The listing builds one solid part. Answer for the finished solid, in the listing's coordinates (mm). Face numbers are marked on the shaded views. A direction names the side the tool comes from. Give positions to 0.01 mm unless a question says otherwise; leave off trailing zeros. Loops run counter-clockwise (first coordinate to the right, second up) from the corner with the lowest first, then second, coordinate; pieces in that order, holes last. Notation, with made-up numbers: M 88,31.5 L 115,31.5 A14 cw 115,49.5 Z; hole C -38,88.25 d9. An arc over 180 degrees is marked long. Return JSON: item names as keys, results as strings.
from build123d import *

# Parameters (mm, degrees)
SKETCH1_R           = 26
BOSS_EXTRUDE1_DEPTH = 60
SKETCH2_R           = 75
SKETCH2_R_2         = 70
CUT_EXTRUDE1_DEPTH  = 20
SKETCH3_R           = 75
SKETCH3_R_2         = 70
CUT_EXTRUDE2_DEPTH  = 20


with BuildPart() as part:
    # Sketch1 → Boss-Extrude1 (new body)
    with BuildSketch(Plane(origin=(0, 0, 0), x_dir=(1, 0, 0), z_dir=(0, 1, 0))):
        with BuildLine():
            Line((-85, 0), (-112.580048144, 0))
            Line((-112.580048144, 0), (-112.580048144, 8.059280082))
            Line((-112.580048144, 8.059280082), (-84.617066863, 8.059280082))
            ThreePointArc((-84.617066863, 8.059280082), (84.904212744, -4.034186201), (-85, 0))
        make_face()
        Circle(SKETCH1_R, mode=Mode.SUBTRACT)
    extrude(amount=BOSS_EXTRUDE1_DEPTH)

    # Sketch2 → Cut-Extrude1 (cut)
    with BuildSketch(Plane(origin=(0, 0, 0), x_dir=(-1, 0, 0), z_dir=(0, -1, 0))):
        Circle(SKETCH2_R)
        Circle(SKETCH2_R_2, mode=Mode.SUBTRACT)
    extrude(amount=-CUT_EXTRUDE1_DEPTH, mode=Mode.SUBTRACT)

    # Sketch3 → Cut-Extrude2 (cut)
    with BuildSketch(Plane(origin=(0, 60, 0), x_dir=(1, 0, 0), z_dir=(0, 1, 0))):
        Circle(SKETCH3_R)
        Circle(SKETCH3_R_2, mode=Mode.SUBTRACT)
    extrude(amount=-CUT_EXTRUDE2_DEPTH, mode=Mode.SUBTRACT)


solid = part.part
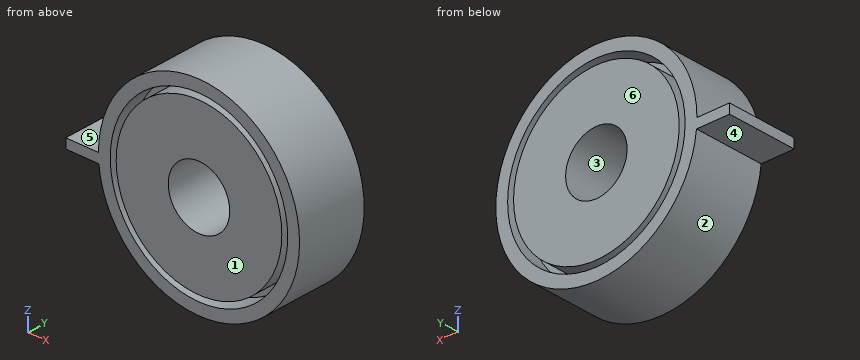
(1) Given pin 1 (2 mm diameter, centred on x = -35.5, y = 30, fed in from -Z); pin 2 (12 mm diameter, centred on y = 34, z = 30, fed in from -X); pin 3 (12 mm diameter, centred on x = 8, z = 16, fed in from +Y); pin 4 (2 mm diameter, centred on y = 47, z = -36.5, fed in from +X), each flat-ended and moving along its own axis, determine where each tip first touches the part or whether it passes through.
Values follow:
{"pin 1": "z = -77.68", "pin 2": "x = -81.54", "pin 3": "through", "pin 4": "x = 77.23"}
(2) The part is cut by section B-B (y = 52.5). Determine the outline of the cut face in (x, z).
Values follow:
{"outline": "M -112.58,-8.06 L -84.62,-8.06 A85 ccw long -85,0 L -112.58,0 Z; C 0,0 d140; hole C 0,0 d150; hole C 0,0 d52"}
(3) Determine the mould class of the marked faces 1, 2 and 3 for opening direction X: released by +X, released by -X, zero draft, split by the parting line, or undercut.
Values follow:
{"face 1": "zero draft", "face 2": "split by the parting line", "face 3": "undercut"}
(4) A tool of negligible diameter and unlimited length cuts with its end or side. For the marked faces 4, 5 and 6, from which of +Z, -Z, +X, -X, +Y, -Y can it reach the whole face along a straight path? Write none if from no direction.
Values follow:
{"face 4": "-Z, -X, +Y, -Y", "face 5": "+Z, -X, +Y, -Y", "face 6": "+Z, -Z, +X, -X, +Y"}
(5) The part is cut by section C-C (y = 23). Determine the outline of the cut face in (x, z), and give its area (3 significant figures).
Values follow:
{"outline": "M -112.58,-8.06 L -84.62,-8.06 A85 ccw long -85,0 L -112.58,0 Z; hole C 0,0 d52", "area": "20,800 mm²"}
(6) The part is cut by section A-A (x = 0). Determine the outline of the cut face in (y, z), and give its area (3 significant figures).
Values follow:
{"outline": "M 0,-85 L 60,-85 L 60,-75 L 40,-75 L 40,-70 L 60,-70 L 60,-26 L 0,-26 L 0,-70 L 20,-70 L 20,-75 L 0,-75 Z; M 0,26 L 60,26 L 60,70 L 40,70 L 40,75 L 60,75 L 60,85 L 0,85 L 0,75 L 20,75 L 20,70 L 0,70 Z", "area": "6,680 mm²"}
(7) Straight lines are drawn through the part: line 1 along Z through (x, y) = (0, 6.5); line 2 along X through (y, z) = (44, -30.5); line 3 along Z through (x, y) = (13.5, 17) (3 decimals). For each, find the intervals that lie inside material, in ascending order.
Values follow:
{"line 1": "-85 to -75, -70 to -26, 26 to 70, 75 to 85", "line 2": "-79.34 to -68.52, -63.01 to 63.01, 68.52 to 79.34", "line 3": "-83.921 to -73.775, -68.686 to -22.22, 22.22 to 68.686, 73.775 to 83.921"}
(8) The part is cut by section D-D (z = 9). Determine the outline of the cut face in (x, y).
Values follow:
{"outline": "M -84.52,0 L -74.46,0 L -74.46,20 L -69.42,20 L -69.42,0 L -24.39,0 L -24.39,60 L -69.42,60 L -69.42,40 L -74.46,40 L -74.46,60 L -84.52,60 Z; M 24.39,0 L 69.42,0 L 69.42,20 L 74.46,20 L 74.46,0 L 84.52,0 L 84.52,60 L 74.46,60 L 74.46,40 L 69.42,40 L 69.42,60 L 24.39,60 Z"}
